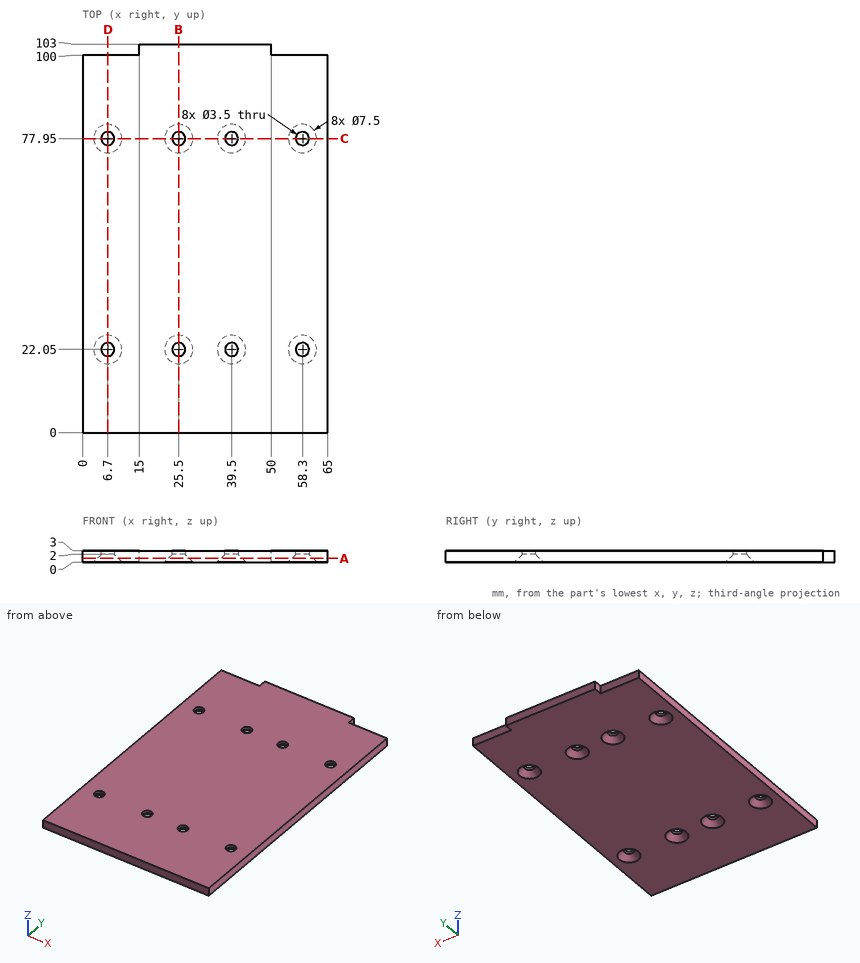
Geometry: see drawing. Coordinates: mm, zero at the bounding-box minimum. Round coordinates to 2 decimals unless told otherwise and drop trailing zeros. Write each loop counter-clockwise with the first axis right and the second up, starting at its lowest first coordinate (ties: lowest second). Pieces come first, ordered by that corner, then holes. Notation, with made-up numbers: (47.25, 3.5) - (103.25, 3.5) arc R19 cw to (103.25, 17.5) - close; hole circle Ø9 at (26.25, 59). An arc over 180 degrees is marked (long way). Use CSV: the item, a comma, the result in double quotes. Start each with the question number.
(1) Cut plane C-C, the plane y = 77.95. Return loops of the section in (x, z).
(2) Cut plane D-D, the plane x = 6.7. Return loops of the section in (y, z), and give its area (3 significant figures).
(3) First-contact query: pin 1 Ø2 at (x, y) = (25.5, 77.95) entering from -Z; pin 2 Ø1.5 at (y, z) = (102, 1.5) entering from -X. Flat tips, straight axial feed; report the tip coordinate or a pass-through.
(4) Material intervals for probe 1 along X at (y, z) = (77.95, 2.65); probe 2 along Y at (x, z) = (58.3, 2.85); probe 3 along Y at (x, z) = (39.5, 2.45), sorted ascending. Write a range as [from, to].
(5) Cut plane B-B, the plane x = 25.5. Return loops of the section in (y, z).
(6) Cut plane A-A, the plane z = 0.95. Give the number of separate pieces and of enclosed holes in the cut face, and give its area (3 significant figures).
Geometry says:
1,outline,"(0, 0) - (2.95, 0) - (4.95, 2) - (4.95, 3) - (0, 3) - close; (8.45, 2) - (10.45, 0) - (21.75, 0) - (23.75, 2) - (23.75, 3) - (8.45, 3) - close; (27.25, 2) - (29.25, 0) - (35.75, 0) - (37.75, 2) - (37.75, 3) - (27.25, 3) - close; (41.25, 2) - (43.25, 0) - (54.55, 0) - (56.55, 2) - (56.55, 3) - (41.25, 3) - close; (60.05, 2) - (62.05, 0) - (65, 0) - (65, 3) - (60.05, 3) - close"
2,outline,"(0, 0) - (18.3, 0) - (20.3, 2) - (20.3, 3) - (0, 3) - close; (23.8, 2) - (25.8, 0) - (74.2, 0) - (76.2, 2) - (76.2, 3) - (23.8, 3) - close; (79.7, 2) - (81.7, 0) - (100, 0) - (100, 3) - (79.7, 3) - close"
2,area,"271 mm²"
3,pin 1,"through"
3,pin 2,"x = 15"
4,probe 1,"[0, 4.95], [8.45, 23.75], [27.25, 37.75], [41.25, 56.55], [60.05, 65]"
4,probe 2,"[0, 20.3], [23.8, 76.2], [79.7, 100]"
4,probe 3,"[0, 20.3], [23.8, 76.2], [79.7, 103]"
5,outline,"(0, 0) - (18.3, 0) - (20.3, 2) - (20.3, 3) - (0, 3) - close; (23.8, 2) - (25.8, 0) - (74.2, 0) - (76.2, 2) - (76.2, 3) - (23.8, 3) - close; (79.7, 2) - (81.7, 0) - (103, 0) - (103, 3) - (79.7, 3) - close"
6,separate pieces,"1"
6,enclosed holes,"8"
6,area,"6,410 mm²"
